from build123d import *
from build123d.topology import SkipClean

# Parameters (mm, degrees)
CUT_EXTRUDE_748_DEPTH      = 70.85
PATTERN_CIRCULAR_802_COUNT = 5
SKETCH_7_R                 = 50
EXTRUDE_1_DEPTH            = 5
CUT_EXTRUDE_START          = -1.6
SKETCH_8_R                 = 50
SKETCH_8_R_2               = 45
CUT_EXTRUDE_1_DEPTH        = 1.6
SKETCH_9_R                 = 6
CUT_EXTRUDE_2_DEPTH        = 97.046863561
SKETCH_10_R                = 4.5
CUT_EXTRUDE_4_DEPTH        = 97.046863561
SKETCH_10_4_R              = 2.2
CUT_EXTRUDE_5_DEPTH        = 8
CHAMFER_1_SIZE             = 0.5
CHAMFER_2_SIZE             = 0.5
CHAMFER_3_SIZE             = 5
EXTRUDE_START              = 7
EXTRUDE_2_DEPTH            = 7
CHAMFER_4_SIZE             = 1
CHAMFER_5_SIZE             = 2
CHAMFER_6_SIZE             = 0.6


with BuildPart() as part:
    # Эскиз2 → Revolve 380 (revolve)
    with BuildSketch(Plane.XY, mode=Mode.PRIVATE) as revolve_380_sk:
        with BuildLine():
            Line((0, 0), (-47.75, 0))
            Line((-47.75, 0), (-47.75, -60))
            Line((-47.75, -60), (-45.75, -60))
            Line((-45.75, -60), (-45.75, -21))
            ThreePointArc((-45.75, -21), (-44.871320344, -18.878679656), (-42.75, -18))
            Line((-42.75, -18), (0, -18))
            Line((0, -18), (0, 0))
        make_face()
    revolve(revolve_380_sk.sketch.rotate(Axis((0, 0, 0), (0, 1, 0)), 270), axis=Axis((0, 0, 0), (0, 1, 0)))

    # Эскиз4 → Cut-Extrude 748 (cut, symmetric)
    with BuildSketch(Plane.XY):
        Polygon((-9, -25), (0, -56.5), (9, -25), align=None)
    cut_extrude_748 = extrude(amount=CUT_EXTRUDE_748_DEPTH, both=True, mode=Mode.SUBTRACT)

    # Pattern Circular 802: Cut-Extrude 748 ×5 about axis
    pattern_circular_802_axis = Axis((0, 0, 0), (0, 1, 0))
    for i in range(1, PATTERN_CIRCULAR_802_COUNT):
        add(cut_extrude_748.rotate(pattern_circular_802_axis, i * 360 / PATTERN_CIRCULAR_802_COUNT), mode=Mode.SUBTRACT)

    # Эскиз7 → Бобышка-Вытянуть1 (add)
    with BuildSketch(Plane(origin=(0, 0, 0), x_dir=(1, 0, 0), z_dir=(0, 1, 0))):
        with Locations(Location((0, 0, 0), (0, 0, 270))):
            Circle(SKETCH_7_R)
    extrude(amount=EXTRUDE_1_DEPTH)

    # Эскиз8 → Вырез-Вытянуть1 (cut)
    with BuildSketch(Plane(origin=(0, 5, 0), x_dir=(1, 0, 0), z_dir=(0, 1, 0)).offset(CUT_EXTRUDE_START)):
        with Locations(Location((0, 0, 0), (0, 0, 270))):
            Circle(SKETCH_8_R)
        with Locations(Location((0, 0, 0), (0, 0, 270))):
            Circle(SKETCH_8_R_2, mode=Mode.SUBTRACT)
    extrude(amount=CUT_EXTRUDE_1_DEPTH, mode=Mode.SUBTRACT)

    # Эскиз9 → Вырез-Вытянуть2 (cut, through all)
    with BuildSketch(Plane(origin=(0, 5, 0), x_dir=(1, 0, 0), z_dir=(0, 1, 0))):
        with Locations(Location((0, 0, 0), (0, 0, 270))):
            Circle(SKETCH_9_R)
    extrude(amount=-CUT_EXTRUDE_2_DEPTH, mode=Mode.SUBTRACT)

    # Эскиз10 → Вырез-Вытянуть4 (cut, through all)
    with BuildSketch(Plane(origin=(0, 5, 0), x_dir=(1, 0, 0), z_dir=(0, 1, 0))):
        with Locations(Location((0, 30, 0), (0, 0, 270))):
            Circle(SKETCH_10_R)
    extrude(amount=-CUT_EXTRUDE_4_DEPTH, mode=Mode.SUBTRACT)

    # Эскиз10<4> → Вырез-Вытянуть5 (cut)
    with BuildSketch(Plane(origin=(0, 5, 0), x_dir=(1, 0, 0), z_dir=(0, 1, 0))):
        with Locations(Location((0, -30, 0), (0, 0, 270))):
            Circle(SKETCH_10_4_R)
        with Locations(Location((-25.980762114, 15, 0), (0, 0, 270))):
            Circle(SKETCH_10_4_R)
        with Locations(Location((25.980762114, 15, 0), (0, 0, 270))):
            Circle(SKETCH_10_4_R)
    extrude(amount=-CUT_EXTRUDE_5_DEPTH, mode=Mode.SUBTRACT)

    # Фаска1
    chamfer_1_edges = [part.edges().sort_by_distance(p)[0] for p in [
        (0, 5, -34.5),
        (-25.980762114, 5, -17.2),
        (25.980762114, 5, -17.2),
        (0, 5, 27.8),
    ]]
    chamfer(chamfer_1_edges, length=CHAMFER_1_SIZE)

    # Фаска2
    chamfer_2_edges = [part.edges().sort_by_distance(p)[0] for p in [
        (0, 5, -6),
    ]]
    chamfer(chamfer_2_edges, length=CHAMFER_2_SIZE)

    # Фаска3
    chamfer_3_edges = [part.edges().sort_by_distance(p)[0] for p in [
        (0, -18, -6),
        (0, -18, -34.5),
    ]]
    chamfer(chamfer_3_edges, length=CHAMFER_3_SIZE)

    # Эскиз13 → Бобышка-Вытянуть2 (add)
    with SkipClean():  # the faces are left unmerged after this step: merging them gives an invalid solid
        with BuildSketch(Plane.XZ.offset(EXTRUDE_START)):
            with BuildLine():
                Line((-1.91, -47.711784708), (-2, -49.959983987))
                ThreePointArc((-2, -49.959983987), (0, -50), (2, -49.959983987))
                Line((2, -49.959983987), (1.91, -47.711784708))
                ThreePointArc((1.91, -47.711784708), (0, -47.75), (-1.91, -47.711784708))
            make_face()
        extrude(amount=-EXTRUDE_2_DEPTH)

    # Фаска4
    chamfer_4_edges = [part.edges().sort_by_distance(p)[0] for p in [
        (1.955, -7, -48.835884347),
        (-1.955, -7, -48.835884347),
    ]]
    chamfer(chamfer_4_edges, length=CHAMFER_4_SIZE)

    # Фаска5
    chamfer_5_edges = [part.edges().sort_by_distance(p)[0] for p in [
        (0, -60, 47.75),
    ]]
    chamfer(chamfer_5_edges, length=CHAMFER_5_SIZE - 0.0001)  # a hair under: the kernel refuses the full size

    # Фаска6
    chamfer_6_edges = [part.edges().sort_by_distance(p)[0] for p in [
        (0, 5, -45),
    ]]
    chamfer(chamfer_6_edges, length=CHAMFER_6_SIZE)


solid = part.part
Part model, mm, in its own coordinate system. A direction names the side the tool comes from. Coordinates: 2 decimals unless noted, no trailing zeros. Write each question's results on one line, items separated by ' | '. Start each with the question number.
Q1. Slice it at B-B on y = -33. Give the number of separate pieces and of enclosed holes in the cut face, and give its area (3 significant figures).
Q2. Drop flat-ended pins along their axis: pin 1 Ø1.3 at (x, z) = (1, 29.5) entering from +Y; pin 2 Ø1 at (x, y) = (-24, -17) entering from +Z; pin 3 Ø8 at (y, z) = (-46.5, 34.5) entering from +X; pin 4 Ø1 at (x, y) = (-2.5, -39.5) entering from -Z. Give the stop position or say it passes through.
Q3. Two-plate mould, pull along Y, no slides. Class faces 4 (the flat face through (45.69, -40.97, -10.18)), 5 (the flat face through (19, 3.4, -41)): +Y half, -Y half, draft (parallel to the pull), parting line (faces both ways), or undercut.
Q4. Probe line 1 along X through (y, z) = (-9, 0); line 2 along Y through (x, z) = (12.5, 6); line 3 along X through (y, z) = (-1.5, -15). List the from-to ranges inside material, lowest first.
Q5. Which spindle directions (+Z, -Z, +X, -X, +Y, -Y) get a long thin tool onto all of the face, cutting with end or side? Do faces 1 (the flat face through (45.733, -40.97, 10.194)), 2 (the flat face through (26, -3, -15)), 3 (the cylindrical face through (-14.343, -29.406, -45.545)). Say none if no direction does.
Answer:
1) separate pieces: 10 | enclosed holes: 0 | area: 318 mm2
2) pin 1: stops at y = -3 | pin 2: stops at z = 41.57 | pin 3: stops at x = 36.74 | pin 4: passes through
3) face 4: undercut | face 5: +Y half
4) line 1: x = -47.75 to -6, 6 to 47.75 | line 2: y = -18 to 5 | line 3: x = -45.33 to -28.18, -23.78 to 23.78, 28.18 to 45.33
5) face 1: none | face 2: +Y | face 3: -Y
